The listing builds one solid part. Answer for the finished solid, in the listing's coordinates (mm). Face numbers are marked on the shaded views. A direction names the side the tool comes from. Give positions to 0.01 mm unless a question says otherwise; leave off trailing zeros. Write each loop counter-clockwise with the first axis right and the second up, starting at its lowest first coordinate (ties: lowest second). Pieces come first, ordered by that corner, then holes.
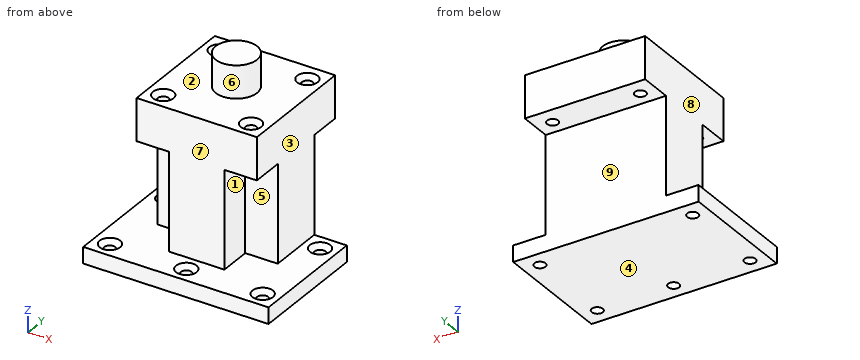
```python
from build123d import *

# Parameters (mm, degrees)
ESQUISSE1_W                                       = 37
ESQUISSE1_H                                       = 37.5
BOSS_EXTRU_1_DEPTH                                = 48
ESQUISSE2_R                                       = 6.375
BOSS_EXTRU_2_DEPTH                                = 10
ENL_V_START                                       = -5
ESQUISSE10_W                                      = 10
ESQUISSE10_H                                      = 10
ESQUISSE10_W_2                                    = 37
ENL_V_MAT_EXTRU_1_DEPTH                           = 30
FRAISAGE_POUR_VIS_T_TE_FRAIS_E_BOMB_E_D           = 3.4
FRAISAGE_POUR_VIS_T_TE_FRAIS_E_BOMB_E_DEPTH       = 13
FRAISAGE_POUR_VIS_T_TE_FRAIS_E_BOMB_E_CSINK_D     = 6.3
FRAISAGE_POUR_VIS_T_TE_FRAIS_E_BOMB_E_CSINK_ANGLE = 90
FRAISAGE_POUR_VIS_T_TE_FRAIS_E_BOMB_E_TIP         = 1.021463052
BOSS_EXTRU_5_DEPTH                                = 5
ESQUISSE12_W                                      = 37
ESQUISSE12_H                                      = 10
ENL_V_MAT_EXTRU_2_DEPTH                           = 5
FRAISAGE_POUR_VIS_T_TE_FRAIS_E_BOM_2_D            = 3.4
FRAISAGE_POUR_VIS_T_TE_FRAIS_E_BOM_2_DEPTH        = 5
FRAISAGE_POUR_VIS_T_TE_FRAIS_E_BOM_2_CSINK_D      = 6.3
FRAISAGE_POUR_VIS_T_TE_FRAIS_E_BOM_2_CSINK_ANGLE  = 90
FRAISAGE_POUR_VIS_T_TE_FRAIS_E_BOM_2_TIP          = 1.021463052


with BuildPart() as part:
    # Esquisse1 → Boss.-Extru.1 (new body)
    with BuildSketch(Plane.XY):
        with Locations((18.5, 18.75)):
            Rectangle(ESQUISSE1_W, ESQUISSE1_H)
    extrude(amount=BOSS_EXTRU_1_DEPTH)

    # Esquisse2 → Boss.-Extru.2 (add)
    with BuildSketch(Plane.XY.offset(48)):
        with Locations((18.5, 19)):
            Circle(ESQUISSE2_R)
    extrude(amount=BOSS_EXTRU_2_DEPTH)

    # Esquisse10 → Enlèv. mat.-Extru.1 (cut)
    with BuildSketch(Plane(origin=(0, 0, 0), x_dir=(-1, 0, 0), z_dir=(0, 0, -1)).offset(ENL_V_START)):
        with Locations((-32, 5)):
            Rectangle(ESQUISSE10_W, ESQUISSE10_H)
        with Locations((-18.5, 32.5)):
            Rectangle(ESQUISSE10_W_2, ESQUISSE10_H)
        with Locations((-5, 5)):
            Rectangle(ESQUISSE10_W, ESQUISSE10_H)
    extrude(amount=-ENL_V_MAT_EXTRU_1_DEPTH, mode=Mode.SUBTRACT)

    # Fraisage pour vis _ t_te frais_e bomb_e
    with Locations(Plane.XY.offset(48)):
        with Locations((5, 32), (32, 32), (32, 5), (5, 5)):
            CounterSinkHole(FRAISAGE_POUR_VIS_T_TE_FRAIS_E_BOMB_E_D / 2, FRAISAGE_POUR_VIS_T_TE_FRAIS_E_BOMB_E_CSINK_D / 2, depth=FRAISAGE_POUR_VIS_T_TE_FRAIS_E_BOMB_E_DEPTH, counter_sink_angle=FRAISAGE_POUR_VIS_T_TE_FRAIS_E_BOMB_E_CSINK_ANGLE)
            with Locations((0, 0, -(FRAISAGE_POUR_VIS_T_TE_FRAIS_E_BOMB_E_DEPTH + FRAISAGE_POUR_VIS_T_TE_FRAIS_E_BOMB_E_TIP / 2))):  # 118° drill point
                Cone(0, FRAISAGE_POUR_VIS_T_TE_FRAIS_E_BOMB_E_D / 2, FRAISAGE_POUR_VIS_T_TE_FRAIS_E_BOMB_E_TIP, mode=Mode.SUBTRACT)

    # Esquisse11 → Boss.-Extru.5 (add)
    with BuildSketch(Plane(origin=(0, 0, 0), x_dir=(-1, 0, 0), z_dir=(0, 0, -1))):
        Polygon((-37, 27.5), (-47, 27.5), (-47, -10), (10, -10), (10, 27.5), (0, 27.5), (0, 0), (-37, 0), align=None)
    extrude(amount=-BOSS_EXTRU_5_DEPTH)

    # Esquisse12 → Enlèv. mat.-Extru.2 (cut)
    with BuildSketch(Plane(origin=(0, 0, 0), x_dir=(-1, 0, 0), z_dir=(0, 0, -1))):
        with Locations((-18.5, 32.5)):
            Rectangle(ESQUISSE12_W, ESQUISSE12_H)
    extrude(amount=-ENL_V_MAT_EXTRU_2_DEPTH, mode=Mode.SUBTRACT)

    # Fraisage pour vis _ t_te frais_e bom 2
    with Locations(Plane.XY.offset(5)):
        with Locations((-5, 22.5), (-5, -5), (18.5, -5), (42, -5), (42, 22.5)):
            CounterSinkHole(FRAISAGE_POUR_VIS_T_TE_FRAIS_E_BOM_2_D / 2, FRAISAGE_POUR_VIS_T_TE_FRAIS_E_BOM_2_CSINK_D / 2, depth=FRAISAGE_POUR_VIS_T_TE_FRAIS_E_BOM_2_DEPTH, counter_sink_angle=FRAISAGE_POUR_VIS_T_TE_FRAIS_E_BOM_2_CSINK_ANGLE)
            with Locations((0, 0, -(FRAISAGE_POUR_VIS_T_TE_FRAIS_E_BOM_2_DEPTH + FRAISAGE_POUR_VIS_T_TE_FRAIS_E_BOM_2_TIP / 2))):  # 118° drill point
                Cone(0, FRAISAGE_POUR_VIS_T_TE_FRAIS_E_BOM_2_D / 2, FRAISAGE_POUR_VIS_T_TE_FRAIS_E_BOM_2_TIP, mode=Mode.SUBTRACT)


solid = part.part
```
Item 1: Each of these flat-tipped pins is pushed along its axis until it touches: P1, Ø11, axis at x = 5, z = 22, coming from the -Y side; P2, Ø1, axis at y = 12.5, z = 42, coming from the +X side; P3, Ø3, axis at y = 17.5, z = 38, coming from the -X side. Where does it stop, or does it pass through?
Conclusion:
P1: stops at y = 0
P2: stops at x = 37
P3: stops at x = 0
Item 2: Consider probe 1 along Y at (x, z) = (5, 41.75); probe 2 along Y at (x, z) = (42, 1.7); probe 3 along X at (y, z) = (5, 41). Determine where each line is inside the solid, lowest interval first.
Conclusion:
probe 1: y = 0 to 3.3, 6.7 to 30.3, 33.7 to 37.5
probe 2: y = -10 to -6.7, -3.3 to 20.8, 24.2 to 27.5
probe 3: x = 0 to 3.3, 6.7 to 30.3, 33.7 to 37
Item 3: A cutting plane is placed at A-A, the plane y = 5. Give the vertices of the cut face in (x, z).
Conclusion:
outline: (-10, 0) - (47, 0) - (47, 5) - (27, 5) - (27, 35) - (30.3, 35) - (30.3, 46.55) - (28.85, 48) - (8.15, 48) - (6.7, 46.55) - (6.7, 35) - (10, 35) - (10, 5) - (-10, 5) - close; (0, 35) - (3.3, 35) - (3.3, 46.55) - (1.85, 48) - (0, 48) - close; (33.7, 35) - (37, 35) - (37, 48) - (35.15, 48) - (33.7, 46.55) - close
Item 4: A cutting plane is placed at C-C, the plane z = 43. Give the vertices of the cut face in (x, y), plus the area to 3 significant figures.
Conclusion:
outline: (0, 0) - (37, 0) - (37, 37.5) - (0, 37.5) - close; hole circle Ø3.4 at (5, 5); hole circle Ø3.4 at (5, 32); hole circle Ø3.4 at (32, 5); hole circle Ø3.4 at (32, 32)
area: 1,350 mm2
Item 5: A cutting plane is placed at D-D, the plane y = -5. Give the vertices of the cut face in (x, z).
Conclusion:
outline: (-10, 0) - (-6.7, 0) - (-6.7, 3.55) - (-8.15, 5) - (-10, 5) - close; (-3.3, 0) - (16.8, 0) - (16.8, 3.55) - (15.35, 5) - (-1.85, 5) - (-3.3, 3.55) - close; (20.2, 0) - (40.3, 0) - (40.3, 3.55) - (38.85, 5) - (21.65, 5) - (20.2, 3.55) - close; (43.7, 0) - (47, 0) - (47, 5) - (45.15, 5) - (43.7, 3.55) - close
Item 6: Determine the mould class of the marked faces 1, 2, 3 and 4 for opening direction Z: pulls with the +Z half, pulls with the -Z half, needs draft (parallel to the pull), parting line crosses it, or undercut.
Conclusion:
face 1: undercut
face 2: pulls with the +Z half
face 3: needs draft
face 4: pulls with the -Z half
Item 7: A cutting plane is placed at B-B, the plane x = -5. Give the vertices of the cut face in (y, z), plus the area to 3 significant figures.
Conclusion:
outline: (-10, 0) - (-6.7, 0) - (-6.7, 3.55) - (-8.15, 5) - (-10, 5) - close; (-3.3, 0) - (20.8, 0) - (20.8, 3.55) - (19.35, 5) - (-1.85, 5) - (-3.3, 3.55) - close; (24.2, 0) - (27.5, 0) - (27.5, 5) - (25.65, 5) - (24.2, 3.55) - close
area: 149 mm2
Item 8: Which of the six approach directions +Z, -Z, +X, -X, +Y, -Y give full straight-line access (tool end or side, diameter ignored) to the marked faces 5, 6, 7, 8 and 9?
Conclusion:
face 5: +X, -Y
face 6: +Z
face 7: +Z, +X, -X, -Y
face 8: +Z, -X, +Y, -Y
face 9: -Z, +X, -X, +Y
